The model under review builds one solid part; all positions refer to its coordinate system, in mm. Face numbers are marked on the shaded views. A direction names the side the tool comes from. Give positions to 0.01 mm unless a question says otherwise; leave off trailing zeros. Order: outer loops, then holes, each group sorted by start corner. A loop starts at its lowest first (then second) coordinate and runs counter-clockwise, first axis right, second up. Notation, with made-up numbers: (30.25, 80) -> (52.25, 80) arc R24 cw to (52.25, 104) -> close; hole circle Ø3 at (35, -1). An arc over 180 degrees is marked (long way). Use one line per item in the form item = value.
```python
from build123d import *

# Parameters (mm, degrees)
SKETCH_2_R           = 15
EXTRUDE_1_REACH      = 155.052
EXTRUDE_1_END_RADIUS = 15
SKETCH_3_R           = 12.5
EXTRUDE_2_REACH      = 208.458
EXTRUDE_2_END_RADIUS = 15
SKETCH_4_R           = 12.5
SHELL_1_T            = -2


with BuildPart() as part:
    # 스윕1: sweep along a path in 스케치1
    with BuildLine(Plane.XY) as sweep_1_path:
        Line((0, 100), (0, 40))
        ThreePointArc((0, 40), (11.715728753, 11.715728753), (40, 0))
        Line((40, 0), (140, 0))
    # 스케치2 → 스윕1 (sweep)
    with BuildSketch(Plane(origin=(140, 0, 0), x_dir=(0, 0, -1), z_dir=(1, 0, 0))):
        Circle(SKETCH_2_R)
    sweep(path=sweep_1_path.line)

    # 보스-돌출1: up to this cylinder (the profile starts outside it)
    extrude_1_end = Plane(origin=(95, 0, 0), z_dir=(1, 0, 0)) * Cylinder(EXTRUDE_1_END_RADIUS, 341.104, mode=Mode.PRIVATE)
    # 스케치3 → 보스-돌출1 (add, up to the surface)
    with BuildSketch(Plane(origin=(0, 40, 0), x_dir=(1, 0, 0), z_dir=(0, 1, 0)), mode=Mode.PRIVATE) as extrude_1_sk1:
        with Locations(Location((95, 0, 0), (0, 0, 270))):
            Circle(SKETCH_3_R)
    extrude_1_tool1 = extrude(extrude_1_sk1.sketch, amount=-EXTRUDE_1_REACH, mode=Mode.PRIVATE) - extrude_1_end
    add(extrude_1_tool1.solids().sort_by_distance((95, 40, 0))[0])

    # 보스-돌출2: up to this cylinder (the profile starts outside it)
    extrude_2_end = Plane(origin=(0, 75, 0), z_dir=(0, -1, 0)) * Cylinder(EXTRUDE_2_END_RADIUS, 447.916, mode=Mode.PRIVATE)
    # 스케치4 → 보스-돌출2 (add, up to the surface)
    with BuildSketch(Plane(origin=(-40, 0, 0), x_dir=(0, 0, -1), z_dir=(1, 0, 0)), mode=Mode.PRIVATE) as extrude_2_sk1:
        with Locations(Location((0, 75, 0), (0, 0, 180))):
            Circle(SKETCH_4_R)
    extrude_2_tool1 = extrude(extrude_2_sk1.sketch, amount=EXTRUDE_2_REACH, mode=Mode.PRIVATE) - extrude_2_end
    add(extrude_2_tool1.solids().sort_by_distance((-40, 75, 0))[0])

    # 쉘1
    shell_1_openings = [part.faces().sort_by_distance(p)[0] for p in [
        (95, 40, 0),
        (-40, 75, 0),
        (140, 0, 0),
        (0, 100, 0),
    ]]
    offset(amount=SHELL_1_T, openings=shell_1_openings, kind=Kind.INTERSECTION)


solid = part.part
```
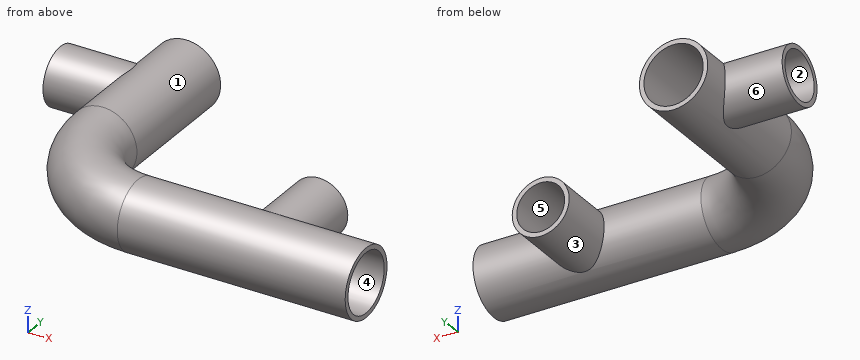
1. Add section A-A on z = 0. Count the separate pieces of the cut face and the enclosed holes in it, then the cut area to 3 significant figures.
Values:
separate_pieces = 4
enclosed_holes = 0
area = 1,010 mm^2
2. For L1, parallel to X at y = 18, z = -11; L2, parallel to Z at x = 48.5, y = 1; L3, parallel to Z at x = -14, y = 75, list the stretches that pass through material, from the lowest coordinate up.
Values:
L1 = -5.12 to -1.45, 15.31 to 19.9, 89.06 to 100.94
L2 = -14.97 to -12.96, 12.96 to 14.97
L3 = -12.5 to -10.5, 10.5 to 12.5
3. Add section C-C on x = 95. Give the boundary of the cut face in (y, z), then the cut area to 3 significant figures.
Values:
outline = (7.66, -10.5) arc R13 cw (long way) to (7.66, 10.5) -> (40, 10.5) -> (40, 12.5) -> (8.29, 12.5) arc R15 ccw (long way) to (8.29, -12.5) -> (40, -12.5) -> (40, -10.5) -> close
area = 250 mm^2
4. Add section B-B on y = 75. Give the boundary of the cut face in (x, z), then the cut area to 3 significant figures.
Values:
outline = (-40, -12.5) -> (-8.29, -12.5) arc R15 ccw (long way) to (-8.29, 12.5) -> (-40, 12.5) -> (-40, 10.5) -> (-7.66, 10.5) arc R13 cw (long way) to (-7.66, -10.5) -> (-40, -10.5) -> close
area = 250 mm^2
5. Add section D-D on x = 121. Give the boundary of the cut face in (y, z), then the cut area to 3 significant figures.
Values:
outline = circle Ø30 at (0, 0); hole circle Ø26 at (0, 0)
area = 176 mm^2
6. The part is to be moulded in two halves that separate along Z. For the marked faces 5 and 6, say which applies: +Z half, -Z half, draft (parallel to the pull), parting line (faces both ways), or undercut.
Values:
face_5 = undercut
face_6 = parting line
7. For pin 1 Ø3 at (x, y) = (-4.5, 55.5) entering from -Z; pin 2 Ø7.5 at (x, z) = (94, 5) entering from +Y; pin 3 Ø12 at (y, z) = (32, 4) entering from +X, all flat-tipped, find the tip position at first contact; note any pin that passes through.
Values:
pin_1 = -14.7
pin_2 = -9.61
pin_3 = 107.5
8. Tool access review of the marked faces 1, 2, 3 and 4: name each direction out of +Z, -Z, +X, -X, +Y, -Y from which nothing blocks a thin tool from reaching the whole face with its end or side.
Values:
face_1 = none
face_2 = -X
face_3 = +Y
face_4 = +X
